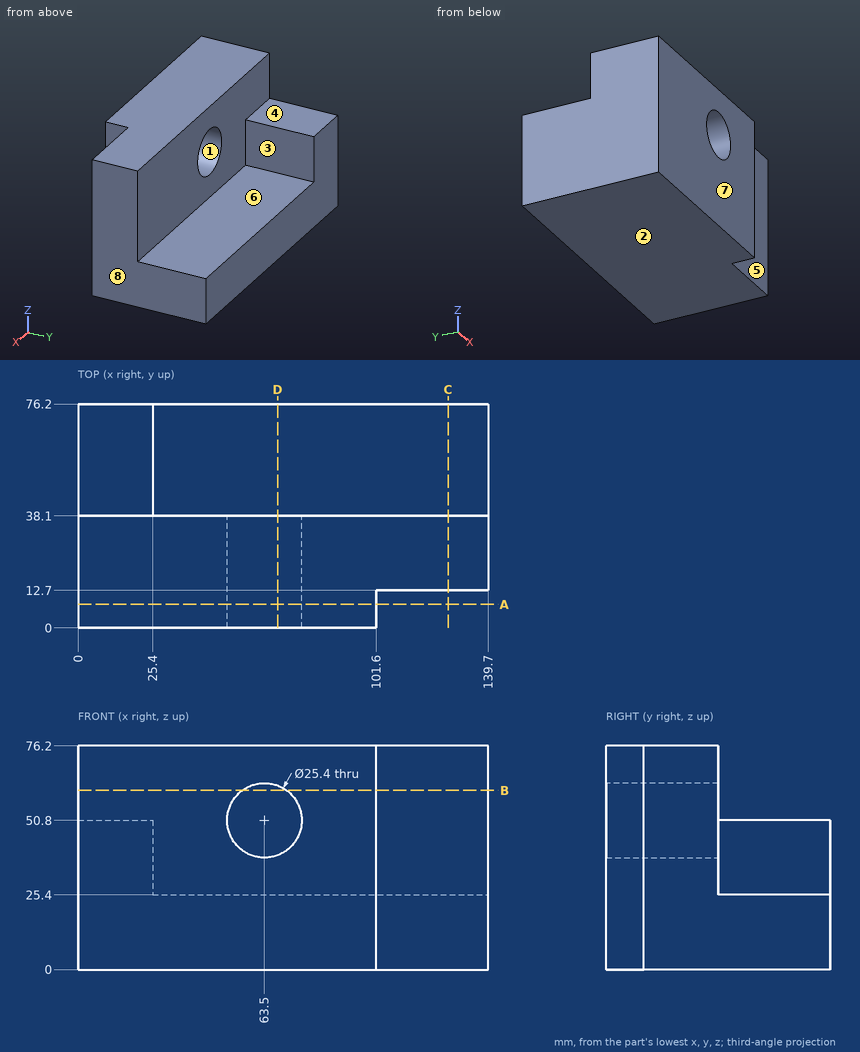
Geometry: see drawing. Coordinates: mm, zero at the bounding-box minimum. A direction names the side the tool comes from. Give positions to 0.01 mm unless a question says otherwise; leave off trailing zeros. Loops run counter-clockwise (first coordinate to the right, second up) from the corner with the lowest first, then second, coordinate; pieces in that order, holes last. Notation, with made-up numbers: (-6, 11) -> (0, 11) arc R25 ccw to (0, 39) -> close; hole circle Ø5 at (-1.5, 44). An arc over 180 degrees is marked (long way). Put each result on its own line as item: value.
1. Set-up query: the marked faces 4, 5, 6, 7 and 8. Return all of +Z, -Z, +X, -X, +Y, -Y with unobstructed straight access to the full face (end or side cutting, diameter ignored); none if empty.
Taken from the geometry:
face 4: +Z, +X, -X, +Y
face 5: +Z, -Z, +X, -Y
face 6: +Z, +X, +Y
face 7: +Z, -Z, +X, -X, -Y
face 8: +Z, -Z, +X, +Y, -Y
2. Pin query (flat end, axial travel): P1, Ø20.5, axis at y = 50, z = 35, coming from the +X side; P2, Ø12.5, axis at x = 19, y = 49, coming from the +Z side; P3, Ø10, axis at y = 5, z = 47.5, coming from the +X side; P4, Ø19, axis at x = 128, z = 23, coming from the -Y side. Return the tip coordinate at first contact, or that it passes through.
Taken from the geometry:
P1: stops at x = 139.7
P2: stops at z = 50.8
P3: stops at x = 101.6
P4: stops at y = 12.7
3. Ray query, line 1 along Z through (x, y) = (63, 11); line 2 along X through (y, z) = (28, 50); line 3 along X through (y, z) = (12, 50). Return the intervals inside material, ascending. Write a range as [from, to].
Taken from the geometry:
line 1: z = [0, 38.11], [63.49, 76.2]
line 2: x = [0, 50.83], [76.17, 139.7]
line 3: x = [0, 50.83], [76.17, 101.6]
4. Cut plane C-C (x = 126). Return the cut outline in (y, z), plus the area to 3 significant figures.
Taken from the geometry:
outline: (12.7, 0) -> (76.2, 0) -> (76.2, 25.4) -> (38.1, 25.4) -> (38.1, 76.2) -> (12.7, 76.2) -> close
area: 2,900 mm2
5. Cut plane A-A (y = 8). Return the cut outline in (x, z), plus the area to 3 significant figures.
Taken from the geometry:
outline: (0, 0) -> (101.6, 0) -> (101.6, 76.2) -> (0, 76.2) -> close; hole circle Ø25.4 at (63.5, 50.8)
area: 7,240 mm2
6. Cut plane D-D (x = 68). Return the cut outline in (y, z), plus the area to 3 significant figures.
Taken from the geometry:
outline: (0, 0) -> (76.2, 0) -> (76.2, 25.4) -> (38.1, 25.4) -> (38.1, 38.92) -> (0, 38.92) -> close; (0, 62.68) -> (38.1, 62.68) -> (38.1, 76.2) -> (0, 76.2) -> close
area: 2,970 mm2
7. Cut plane B-B (z = 61). Return the cut outline in (x, y), plus the area to 3 significant figures.
Taken from the geometry:
outline: (0, 0) -> (55.93, 0) -> (55.93, 38.1) -> (0, 38.1) -> close; (71.07, 0) -> (101.6, 0) -> (101.6, 12.7) -> (139.7, 12.7) -> (139.7, 38.1) -> (71.07, 38.1) -> close
area: 4,260 mm2
8. Pull-direction query (X, two-part tool) for the marked faces 1, 2 and 3; classes: released by +X, released by -X, zero draft, split by the parting line, or undercut.
Taken from the geometry:
face 1: undercut
face 2: zero draft
face 3: released by +X
